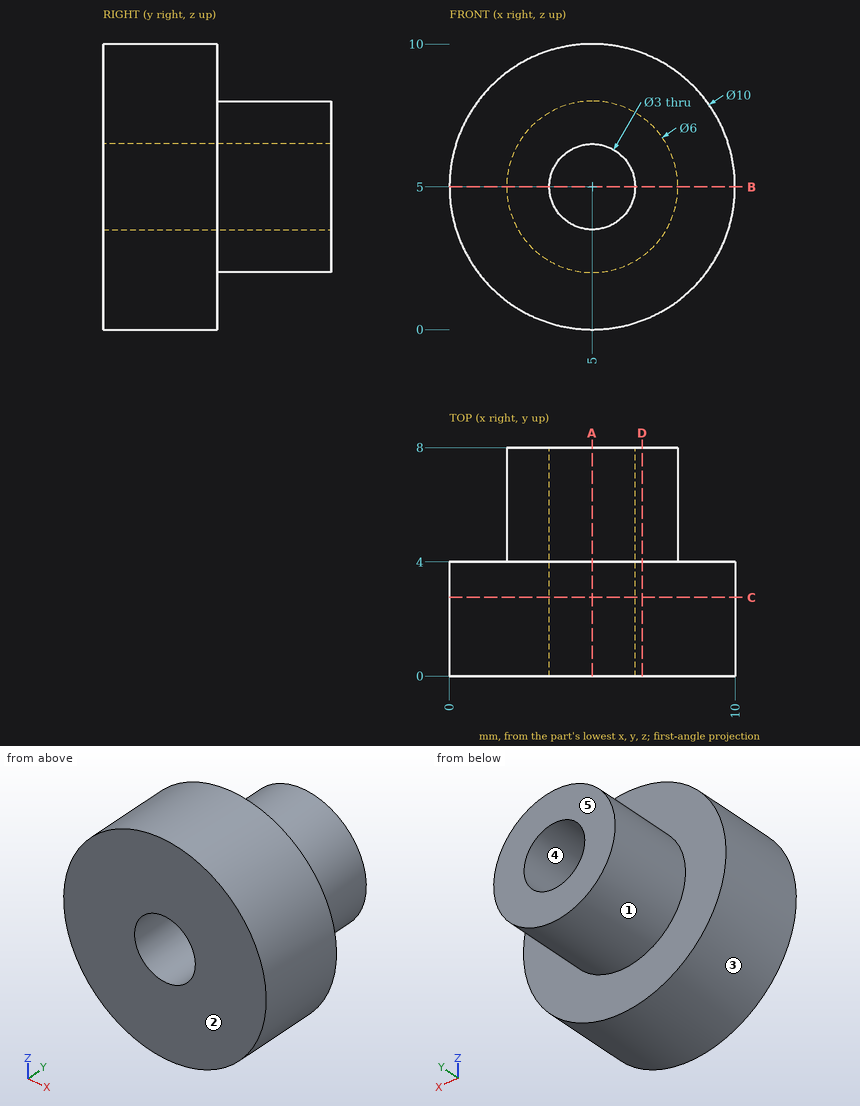
Source: three-view drawing plus pictorial views. Frame: mm from the lowest corner of the part. A direction names the side the tool comes from. Coordinates: 2 decimals unless noted, no trailing zeros. Write each loop counter-clockwise with the first axis right and the second up, starting at its lowest first coordinate (ties: lowest second). Pieces come first, ordered by that corner, then holes. Notation, with made-up numbers: (80.25, 87.5) - (114.25, 87.5) arc R23 ccw to (114.25, 112.5) - close; hole circle Ø9 at (-0.75, -4). An arc over 180 degrees is marked (long way). Return JSON: item names as keys, results as strings.
Item 1: Reachability of the marked faces 1 and 2 from +Z, -Z, +X, -X, +Y, -Y: full face, straight path, thin tool, end or side. Return the list, or none.
Completed:
{"face 1": "+Y", "face 2": "+Z, -Z, +X, -X, -Y"}
Item 2: Section query A-A (x = 5). Output: boundary loops of the cut face in (y, z), and give its area (3 significant figures).
Completed:
{"outline": "(0, 0) - (4, 0) - (4, 2) - (8, 2) - (8, 3.5) - (0, 3.5) - close; (0, 6.5) - (8, 6.5) - (8, 8) - (4, 8) - (4, 10) - (0, 10) - close", "area": "40.0 mm2"}
Item 3: Section query D-D (x = 6.75). Output: boundary loops of the cut face in (y, z).
Completed:
{"outline": "(0, 0.32) - (4, 0.32) - (4, 2.56) - (8, 2.56) - (8, 7.44) - (4, 7.44) - (4, 9.68) - (0, 9.68) - close"}
Item 4: Pin query (flat end, axial travel): pin 1 Ø4 at (x, y) = (2.5, 3) entering from +Z; pin 2 Ø1.5 at (x, y) = (3, 6) entering from -Z. Return the tip coordinate at first contact, or that it passes through.
Completed:
{"pin 1": "stops at z = 9.97", "pin 2": "stops at z = 2.27"}
Item 5: Line query: L1, parallel to X at y = 3.5, z = 5; L2, parallel to X at y = 6.25, z = 5; L3, parallel to Z at x = 4, y = 5.25. Output: solid intervals per line, ascending.
Completed:
{"L1": "x = 0 to 3.5, 6.5 to 10", "L2": "x = 2 to 3.5, 6.5 to 8", "L3": "z = 2.17 to 3.88, 6.12 to 7.83"}
Item 6: Section query C-C (y = 2.75). Output: boundary loops of the cut face in (x, z).
Completed:
{"outline": "circle Ø10 at (5, 5); hole circle Ø3 at (5, 5)"}
Item 7: Pull-direction query (X, two-part tool) for the marked faces 3, 4 and 5; classes: +X half, -X half, draft (parallel to the pull), parting line (faces both ways), or undercut.
Completed:
{"face 3": "parting line", "face 4": "undercut", "face 5": "draft"}
Item 8: Section query B-B (z = 5). Output: boundary loops of the cut face in (x, y).
Completed:
{"outline": "(0, 0) - (3.5, 0) - (3.5, 8) - (2, 8) - (2, 4) - (0, 4) - close; (6.5, 0) - (10, 0) - (10, 4) - (8, 4) - (8, 8) - (6.5, 8) - close"}
